The model under review builds one solid part; all positions refer to its coordinate system, in mm. Coordinates: 2 decimals unless noted, no trailing zeros. Write each loop counter-clockwise with the first axis right and the second up, starting at its lowest first coordinate (ties: lowest second). Pieces come first, ordered by that corner, then holes.
```python
from build123d import *

# Parameters (mm, degrees)
SKETCH_1_W      = 6.1
SKETCH_1_H      = 3.7
EXTRUDE_1_DEPTH = 1.8
SKETCH_3_W      = 2.7
SKETCH_3_H      = 1.3
EXTRUDE_2_DEPTH = 0.7
EXTRUDE_START   = -0.1
SKETCH_4_W      = 1
SKETCH_4_H      = 0.6
EXTRUDE_3_DEPTH = 0.15
FILLET_1_R      = 0.2
FILLET_2_R      = 0.2


with BuildPart() as part:
    # Эскиз1 → Бобышка-Вытянуть1 (new body)
    with BuildSketch(Plane(origin=(0, 0, 0), x_dir=(1, 0, 0), z_dir=(0, 1, 0))):
        Rectangle(SKETCH_1_W, SKETCH_1_H)
    extrude(amount=EXTRUDE_1_DEPTH)

    # Эскиз3 → Бобышка-Вытянуть2 (add)
    with BuildSketch(Plane(origin=(0, 1.8, 0), x_dir=(1, 0, 0), z_dir=(0, 1, 0))):
        Rectangle(SKETCH_3_W, SKETCH_3_H)
    extrude(amount=EXTRUDE_2_DEPTH)

    # Эскиз4 → Бобышка-Вытянуть3 (add)
    with BuildSketch(Plane.XZ.offset(EXTRUDE_START)):
        with Locations((-3.55, 0)):
            Rectangle(SKETCH_4_W, SKETCH_4_H)
    extrude_3 = extrude(amount=EXTRUDE_3_DEPTH)

    # Зеркальное отражение1: Бобышка-Вытянуть3 across plane
    add(extrude_3.mirror(Plane(origin=(0, 0, 0), x_dir=(0, 0, 1), z_dir=(1, 0, 0))))

    # Скругление1
    fillet_1_edges = [part.edges().sort_by_distance(p)[0] for p in [
        (1.35, 2.15, 0.65),
        (1.35, 2.15, -0.65),
        (-1.35, 2.15, -0.65),
        (-1.35, 2.15, 0.65),
    ]]
    fillet(fillet_1_edges, radius=FILLET_1_R)

    # Скругление2
    fillet_2_edges = [part.edges().sort_by_distance(p)[0] for p in [
        (3.05, 0.9, 1.85),
        (-3.05, 0.9, 1.85),
        (-3.05, 0.9, -1.85),
        (3.05, 0.9, -1.85),
    ]]
    fillet(fillet_2_edges, radius=FILLET_2_R)


solid = part.part
```
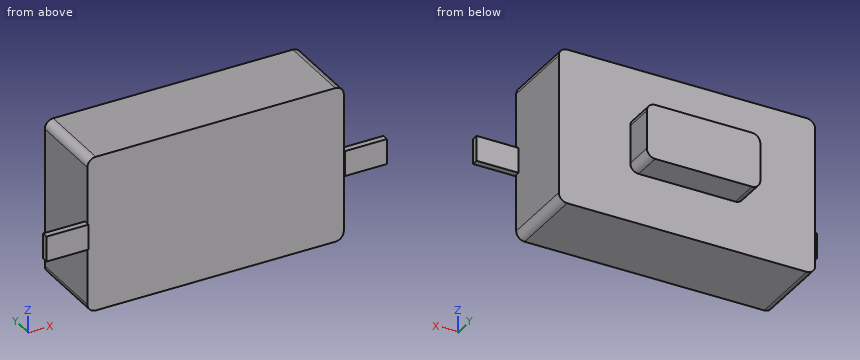
Item 1: For pin 1 (0.7 mm diameter, centred on x = -3.5, z = 0, fed in from +Y); pin 2 (0.5 mm diameter, centred on y = 0.5, z = 0, fed in from +X); pin 3 (1.4 mm diameter, centred on y = 1.5, z = 0.5, fed in from -X), all flat-tipped, find the tip position at first contact; note any pin that passes through.
Solved:
pin 1: stops at y = 0.1
pin 2: stops at x = 3.05
pin 3: stops at x = -3.05
Item 2: To check wall thickness, follow line 1 along X through (y, z) = (0.65, -0.9); line 2 along Y through (x, z) = (0.75, 1.25); line 3 along Z through (x, y) = (1, 2.4). State the ranges of each line that lie inside material, in increasing order.
Solved:
line 1: x = -3.05 to 3.05
line 2: y = 0 to 1.8
line 3: z = -0.65 to 0.65
Item 3: Take a section at D-D, the plane x = -1.5. Write out the cut boundary in (y, z).
Solved:
outline: (0, -1.85) - (1.8, -1.85) - (1.8, 1.85) - (0, 1.85) - close
Item 4: Take a section at A-A, the plane x = -0.5. Write out the cut boundary in (y, z).
Solved:
outline: (0, -1.85) - (1.8, -1.85) - (1.8, -0.65) - (2.5, -0.65) - (2.5, 0.65) - (1.8, 0.65) - (1.8, 1.85) - (0, 1.85) - close
Item 5: Take a section at C-C, the plane y = 1.6. Write out the cut boundary in (x, z), plus the area to 3 significant figures.
Solved:
outline: (-3.05, -1.65) arc R0.2 ccw to (-2.85, -1.85) - (2.85, -1.85) arc R0.2 ccw to (3.05, -1.65) - (3.05, 1.65) arc R0.2 ccw to (2.85, 1.85) - (-2.85, 1.85) arc R0.2 ccw to (-3.05, 1.65) - close
area: 22.5 mm2
Item 6: Take a section at B-B, the plane z = 0.2. Write out the cut boundary in (x, y).
Solved:
outline: (-4.05, -0.05) - (-3.05, -0.05) - (-3.05, 0) - (3.05, 0) - (3.05, -0.05) - (4.05, -0.05) - (4.05, 0.1) - (3.05, 0.1) - (3.05, 1.8) - (1.35, 1.8) - (1.35, 2.5) - (-1.35, 2.5) - (-1.35, 1.8) - (-3.05, 1.8) - (-3.05, 0.1) - (-4.05, 0.1) - close
